Geometry check sheet. Reference: the model listing, model coordinates, mm. A direction names the side the tool comes from. Round coordinates to 2 decimals unless told otherwise and drop trailing zeros. Order: outer loops, then holes, each group sorted by start corner. A loop starts at its lowest first (then second) coordinate and runs counter-clockwise, first axis right, second up.
(1) Draft check along Y on faces 1 (the face through (0, 5, 30)), 2 (the face through (19, 0, 10)), 3 (the face through (-17, 0, 22)). Enter one of: pulls with the +Y half, pulls with the -Y half, needs draft (parallel to the pull), parting line crosses it, or undercut.
(2) Thickness scan on L1, parallel to Y at x = -14.5, z = 27; L2, parallel to Y at x = 13, z = 24.5; L3, parallel to Y at x = 21, z = 11. Record the ranges inside material, lowest first.
(3) Cross-section at A-A on z = 25.5. Enter the section's corners in (x, y), and give its area (3 significant figures).
(4) Set-up check for faces 4 (the face through (-11.014, -10.14, 15.703)), 5 (the face through (-25, 4, 11)), 6 (the face through (10, 0, 20)): record each of +Z, -Z, +X, -X, +Y, -Y from which the full face is reachable in a straight line by a thin tool's end or side.
(5) Gauge pin test, flat ends, axial feed: P1, Ø6, axis at x = -14.5, z = 22.5, coming from the -Y side; P2, Ø4.5, axis at x = 21, y = 7, coming from the +Z side; P3, Ø12, axis at x = -13, y = -11.5, coming from the +Z side. Record the tip position at first contact, or that the pin passes through.
(6) Cross-section at D-D on x = -18.5. Enter the section's corners in (y, z).
(7) Cross-section at C-C on y = 1.5. Enter the section's corners in (x, z), and give its area (3 significant figures).
(8) Cross-section at B-B on x = 14. Enter the section's corners in (y, z), and give its area (3 significant figures).
from build123d import *

# Parameters (mm, degrees)
F0_W     = 50
F0_H     = 40
F1_DEPTH = 30
F2_R     = 20
F3_DEPTH = 20
F4_R     = 15
F5_DEPTH = 20


with BuildPart() as f1:
    # F0 (on Top) → F1 (new body)
    with BuildSketch(Plane.XY):
        Rectangle(F0_W, F0_H)
    extrude(amount=F1_DEPTH)

    # F2 (on face) → F3 (cut)
    with BuildSketch(Plane.XZ.offset(20)):
        with Locations((-25, 30)):
            Circle(F2_R)
    extrude(amount=-F3_DEPTH, mode=Mode.SUBTRACT)

    # F4 (on face) → F5 (cut)
    with BuildSketch(Plane.XY.offset(30)):
        with Locations((25, 0)):
            Circle(F4_R)
    extrude(amount=-F5_DEPTH, mode=Mode.SUBTRACT)


solid = f1.part
Found:
1. face 1: needs draft
1. face 2: undercut
1. face 3: pulls with the -Y half
2. L1: y = 0 to 20
2. L2: y = -20 to -9, 9 to 20
2. L3: y = -20 to -14.46, 14.46 to 20
3. outline: (-25, 0) - (-5.51, 0) - (-5.51, -20) - (25, -20) - (25, -15) arc R15 cw to (25, 15) - (25, 20) - (-25, 20) - close
3. area: 1,260 mm2
4. face 4: +Z, -X, -Y
4. face 5: +Z, -Z, -X, +Y, -Y
4. face 6: +Z, +X
5. P1: stops at y = 0
5. P2: stops at z = 10
5. P3: stops at z = 21.28
6. outline: (-20, 0) - (20, 0) - (20, 30) - (0, 30) - (0, 11.09) - (-20, 11.09) - close
7. outline: (-25, 0) - (25, 0) - (25, 10) - (10.08, 10) - (10.08, 30) - (-25, 30) - close
7. area: 1,200 mm2
8. outline: (-20, 0) - (20, 0) - (20, 30) - (10.2, 30) - (10.2, 10) - (-10.2, 10) - (-10.2, 30) - (-20, 30) - close
8. area: 792 mm2
